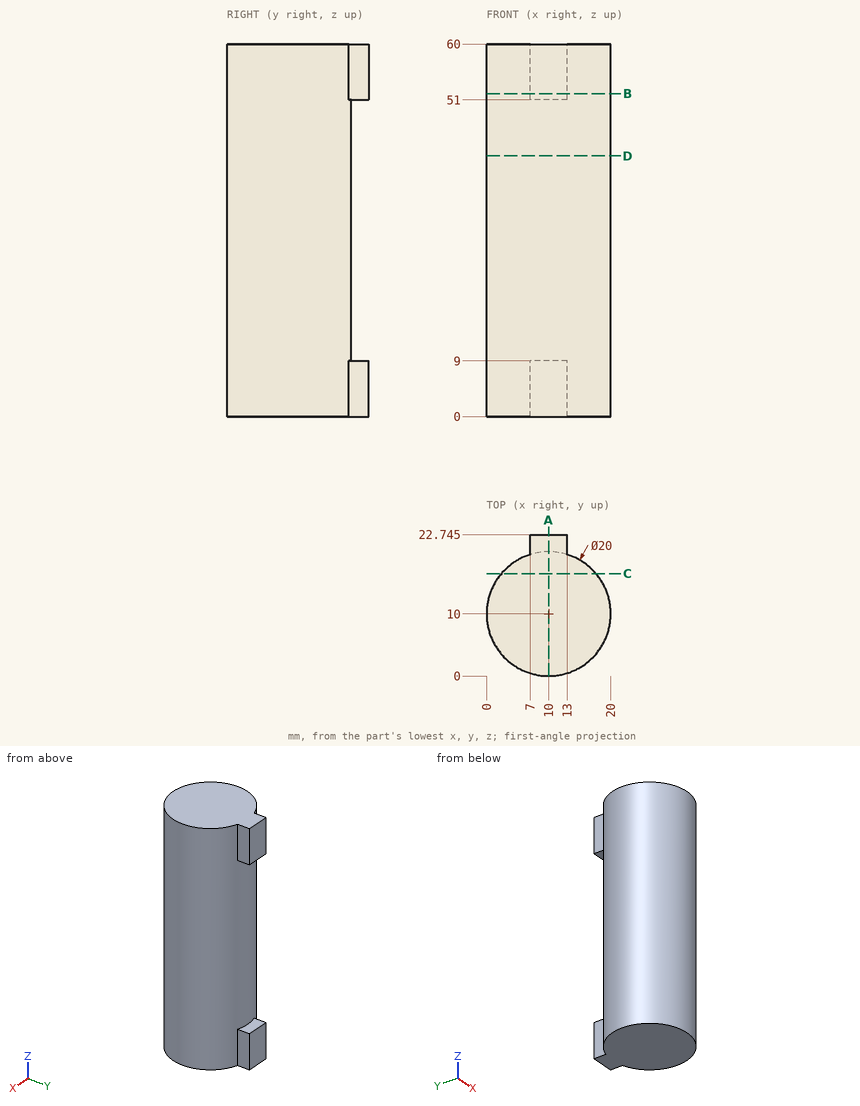
The drawing under review shows one solid part. Ordinate dimensions are in mm from its lowest x, y, z. Coordinates: 2 decimals unless noted, no trailing zeros. Loops run counter-clockwise (first coordinate to the right, second up) from the corner with the lowest first, then second, coordinate; pieces in that order, holes last. Notation, with made-up numbers: (42.5, -5) - (59.5, -5) arc R28 cw to (59.5, 22) - close; hole circle Ø7 at (70.5, -25). An arc over 180 degrees is marked (long way). Return JSON: item names as keys, results as strings.
Item 1: Take a section at C-C (y = 16.5). Give the boundary of the cut face in (x, z), then the cut area to 3 significant figures.
Determined:
{"outline": "(2.4, 0) - (17.6, 0) - (17.6, 60) - (2.4, 60) - close", "area": "912 mm2"}
Item 2: Take a section at A-A (x = 10). Give the boundary of the cut face in (y, z) (3 decimals), then the cut area to 3 significant figures.
Determined:
{"outline": "(0, 0) - (22.745, 0) - (22.745, 9) - (20, 9) - (20, 51) - (22.745, 51) - (22.745, 60) - (0, 60) - close", "area": "1,250 mm2"}
Item 3: Take a section at B-B (z = 52). Give the boundary of the cut face in (x, y) (3 decimals), then the cut area to 3 significant figures.
Determined:
{"outline": "(7, 19.539) arc R10 ccw (long way) to (13, 19.539) - (13, 22.745) - (7, 22.745) - close", "area": "332 mm2"}
Item 4: Take a section at D-D (z = 42). Give the boundary of the cut face in (x, y).
Determined:
{"outline": "circle Ø20 at (10, 10)"}
Item 5: Insertion check: pin 1 (3 mm diameter, centred on x = 3, z = 12.5, fed in from -Y); pin 2 (3 mm diameter, centred on x = 16, z = 14.5, fed in from -Y); pin 3 (12 mm diameter, centred on x = 4.5, z = 30, fed in from +Y). Each pin has a flat end and moves straight along its axis. Give the tip position at first contact, or say it passes through.
Determined:
{"pin 1": "stops at y = 1.65", "pin 2": "stops at y = 1.07", "pin 3": "stops at y = 20"}
Item 6: For line 1 (Z direction, x = 9, y = 21.25); line 2 (X direction, y = 9.5, z = 27.5); line 3 (X direction, y = 21.75, z = 8), list the stretches that pass through material, from the lowest coordinate up.
Determined:
{"line 1": "z = 0 to 9, 51 to 60", "line 2": "x = 0.01 to 19.99", "line 3": "x = 7 to 13"}
